Work out the finished part from the listing and answer in its coordinate system (mm). Face numbers are marked on the shaded views. A direction names the side the tool comes from. Coordinates: 2 decimals unless noted, no trailing zeros. Order: outer loops, then holes, each group sorted by start corner. A loop starts at its lowest first (then second) coordinate and runs counter-clockwise, first axis right, second up.
1. Find the intervals of material crossed by probe 1 along Z at (x, y) = (-3.25, 4.25); probe 2 along Y at (x, z) = (-2, 45.5); probe 3 along Y at (x, z) = (0, 69.5), in increasing order.
2. The part is cut by section A-A, the plane y = 0. Give the vertices of the cut face in (x, z).
3. A tool of negligible diameter and unlimited length cuts with its end or side. For the marked faces 1 and 2, from which of +Z, -Z, +X, -X, +Y, -Y can it reach the whole face along a straight path? Write none if from no direction.
4. Flat-ended cylindrical pins translate along their axes: pin 1 Ø2 at (y, z) = (-2, 56.5) entering from +X; pin 2 Ø1.5 at (y, z) = (4, 20.5) entering from +X; pin 3 Ø5 at (y, z) = (-4.5, 26) entering from +X. Find the tip coordinate at first contact, or state that the pin passes through.
5. The part is cut by section B-B, the plane z = 39. Give the vertices of the cut face in (x, y).
Autodesk Inventor part; units mm, degrees
ref_plane "YZ Plane" through (0, 0, 0) normal (1, 0, 0) x (0, 1, 0)
ref_plane "XZ Plane" through (0, 0, 0) normal (0, 1, 0) x (-1, 0, 0)
ref_plane "XY Plane" through (0, 0, 0) normal (0, 0, 1) x (1, 0, 0)
sketch "Sketch1" plane through (0, 0, 0) normal (0, 0, 1) x (1, 0, 0)
  circle A0 centre (0, 0) radius 4
  dimension "Diameter" = 8
extrude "Extrusion1" add sketch "Sketch1" along normal blind 75
sketch "Sketch2" plane through (0, 0, 75) normal (0, 0, 1) x (1, 0, 0)
  circle A0 centre (0, 0) radius 4
  circle A1 centre (0, 0) radius 6.5
  dimension "Head_Diameter" = 13
extrude "Extrusion2" add sketch "Sketch2" along normal blind 8 contours A0 | A1
sketch "Sketch3" plane through (0, 0, 83) normal (0, 0, 1) x (1, 0, 0)
  circle A0 centre (0, 0) radius 6.5
  circle A1 centre (0, 0) radius 3.4641 construction
  line L0 (0, 3.4641) -> (3, 1.7321)
  line L1 (3, -1.7321) -> (3, 1.7321)
  line L2 (0, 3.4641) -> (-3, 1.7321)
  line L3 (-3, -1.7321) -> (-3, 1.7321)
  line L4 (-3, -1.7321) -> (0, -3.4641)
  line L5 (3, -1.7321) -> (0, -3.4641)
  dimension "Hex_Width" = 6
extrude "Extrusion3" cut sketch "Sketch3" against normal blind 4 contours L0 L1 L5 L4 L3 L2
thread "Thread1"
chamfer "Chamfer1" distance 0.8 angle 45 2 edges at (-6.5, 0, 83) (-4, 0, 0)
equation "\"d9\" = ThreadLength"
equation "\"d12\" = Chamfer"
equation "\"ThreadLength\" = 28"
properties part number "SCREW, SOCKET HD, P, 12_9, M8X1_25X75MM" material "Steel, MS"
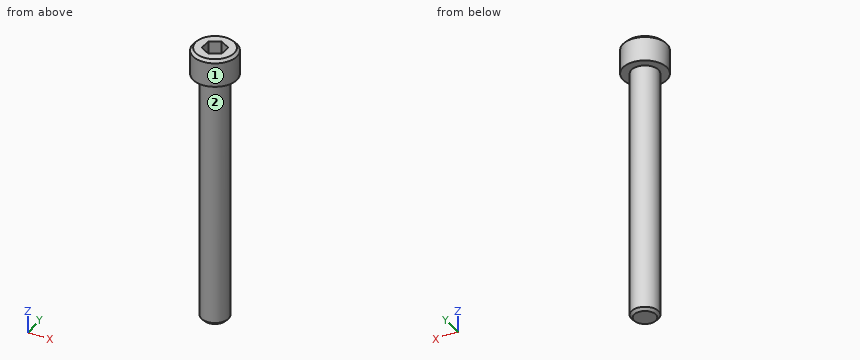
Geometry says:
1. probe 1: z = 75 to 83
1. probe 2: y = -3.46 to 3.46
1. probe 3: y = -4 to 4
2. outline: (-6.5, 75) - (-4, 75) - (-4, 0.8) - (-3.2, 0) - (3.2, 0) - (4, 0.8) - (4, 75) - (6.5, 75) - (6.5, 82.2) - (5.7, 83) - (3, 83) - (3, 79) - (-3, 79) - (-3, 83) - (-5.7, 83) - (-6.5, 82.2) - close
3. face 1: +Z, -Z
3. face 2: -Z
4. pin 1: stops at x = 3.87
4. pin 2: stops at x = 2.33
4. pin 3: stops at x = 3.46
5. outline: circle Ø8 at (0, 0)
